Geometry check sheet. Reference: the model listing, model coordinates, mm. Round coordinates to 2 decimals unless told otherwise and drop trailing zeros. Order: outer loops, then holes, each group sorted by start corner. A loop starts at its lowest first (then second) coordinate and runs counter-clockwise, first axis right, second up. Notation, with made-up numbers: M 45,73 L 72,73 A27 ccw 72,99 Z; hole C -32.75,17.5 d5. An arc over 180 degrees is marked long. Return JSON: item names as keys, results as strings. Group by question number.
```python
from build123d import *

# Parameters (mm, degrees)
EXTRUDE_THIN1_DEPTH          = 107.95
F_3_8_0_375_DIAMETER_HOLE1_D = 9.525


with BuildPart() as part:
    # Sketch1 → Extrude-Thin1 (new, symmetric)
    with BuildSketch(Plane(origin=(0, 0, 0), x_dir=(0, 0, -1), z_dir=(1, 0, 0))):
        Polygon((-38.1, 0), (0, 0), (0, 38.1), (-6.35, 38.1), (-6.35, 6.35), (-38.1, 6.35), align=None)
    extrude(amount=EXTRUDE_THIN1_DEPTH, both=True)

    # 3/8 (0.375) Diameter Hole1 (through all)
    with Locations(Plane.XY.offset(6.35)):
        with Locations((-85.725, 25.4), (85.725, 25.4)):
            Hole(F_3_8_0_375_DIAMETER_HOLE1_D / 2)


solid = part.part
```
Q1. Release check for a two-part mould opening along Y. For faces 1 (the face through (81.182, 26.831, 3.131)), 2 (the face through (2, 6.35, 22)), 3 (the face through (2, 22, 6.35)) record: +Y half, -Y half, draft (parallel to the pull), parting line (faces both ways), or undercut.
Q2. Section check B-B on x = 52. Record the cut outline in (y, z).
Q3. Section check C-C on x = 86. Record the cut outline in (y, z).
Q4. Depth check by flat-ended pin: pin 1 Ø9.5 at (x, z) = (-30.5, 23) entering from +Y; pin 2 Ø16 at (x, y) = (29.5, 21.5) entering from +Z; pin 3 Ø4 at (y, z) = (28, 9.5) entering from -X. Enter the tip coordinate at first touch or a pass-through.
Q5. Section check A-A on y = 25.4. Record the cut outline in (x, z), plus the area to 3 significant figures.
Q6. Section check D-D on y = 13. Record the cut outline in (x, z), plus the area to 3 significant figures.
Q7. Material ranges on line 1 along X through (y, z) = (25, 4); line 2 along Z through (x, y) = (-55, 31.5), recorded low to high.
Geometry check:
{
 "1": {"face 1": "undercut", "face 2": "+Y half", "face 3": "draft"},
 "2": {"outline": "M 0,0 L 38.1,0 L 38.1,6.35 L 6.35,6.35 L 6.35,38.1 L 0,38.1 Z"},
 "3": {"outline": "M 0,0 L 20.65,0 L 20.65,6.35 L 6.35,6.35 L 6.35,38.1 L 0,38.1 Z; M 30.15,0 L 38.1,0 L 38.1,6.35 L 30.15,6.35 Z"},
 "4": {"pin 1": "stops at y = 6.35", "pin 2": "stops at z = 6.35", "pin 3": "passes through"},
 "5": {"outline": "M -107.95,0 L -90.49,0 L -90.49,6.35 L -107.95,6.35 Z; M -80.96,0 L 80.96,0 L 80.96,6.35 L -80.96,6.35 Z; M 90.49,0 L 107.95,0 L 107.95,6.35 L 90.49,6.35 Z", "area": "1,250 mm^2"},
 "6": {"outline": "M -107.95,0 L 107.95,0 L 107.95,6.35 L -107.95,6.35 Z", "area": "1,370 mm^2"},
 "7": {"line 1": "x = -107.95 to -90.47, -80.98 to 80.98, 90.47 to 107.95", "line 2": "z = 0 to 6.35"}
}
